Work out the finished part from the listing and answer in its coordinate system (mm). A direction names the side the tool comes from. Coordinates: 2 decimals unless noted, no trailing zeros. Write each loop counter-clockwise with the first axis right and the second up, starting at its lowest first coordinate (ties: lowest second). Pieces come first, ordered by that corner, then holes. Notation, with made-up numbers: M 61.25,-11.5 L 100.25,-11.5 A38 cw 100.25,26.5 Z; hole C -3.75,11 d2. An arc over 180 degrees is marked long. Answer as CSV lines item,"result". Start each with the question number.
(1) A cutting plane is placed at B-B on z = -9. Give the vertices of the cut face in (x, y) (3 decimals).
(2) Find the intervals of material crossed by L1, parallel to Z at x = -135.5, y = 0.95 (3 decimals); L2, parallel to Z at x = -122.5, y = 0.25 (3 decimals); L3, parallel to X at y = 0.85, z = -173, in increasing order. Write a range as [from, to].
(3) A cutting plane is placed at D-D on y = 1.25. Count the separate pieces of the cut face and the enclosed holes in it, then the cut area to 3 significant figures.
(4) A cutting plane is placed at A-A on x = -135.5. Give the vertices of the cut face in (y, z) (3 decimals), then the cut area to 3 significant figures.
(5) The mould has two halves that part along X. Classify faces 1 (the cylindrical face through (-119.578, 0.74, -9.129)), 2 (the cylindrical face through (-135.12, 0.74, -180.4)), 3 (the cylindrical face through (-115.304, 0.76, -1.711)), 4 (the cylindrical face through (-142.696, 0.76, -202.789)): released by +X, released by -X, zero draft, split by the parting line, or undercut.
(6) A cutting plane is placed at C-C on x = -116.5. Give the vertices of the cut face in (y, z).
(7) For faces 5 (the cylindrical face through (-132.578, 0.74, -27.129)), 6 (the cylindrical face through (-115.211, 0.76, -16.196)), determine the directions among +Z, -Z, +X, -X, +Y, -Y from which every point of the face is accessible in a straight line to the end or side of a thin tool.
(8) A flat-ended cylindrical pin translates along its axis: P1, Ø7.5, axis at x = -122.5, z = -195.5, coming from the +Y side. Find the tip coordinate at first contact, or state that the pin passes through.
Autodesk Inventor part; units mm, degrees
ref_plane "YZ Plane" through (0, 0, 0) normal (1, 0, 0) x (0, 1, 0)
ref_plane "XZ Plane" through (0, 0, 0) normal (0, 1, 0) x (-1, 0, 0)
ref_plane "XY Plane" through (0, 0, 0) normal (0, 0, 1) x (1, 0, 0)
sketch "Sketch1" plane through (0, 0, 0) normal (0, 1, 0) x (-1, 0, 0)
  line L0 (0, 0) -> (144.5, 0) construction
  line L1 (144.5, 0) -> (144.5, -204.5) construction
  line L2 (144.5, -204.5) -> (0, -204.5) construction
  line L3 (0, -204.5) -> (0, 0) construction
  circle A0 centre (135.5, -27) radius 3 construction
  circle A1 centre (122.5, -9) radius 3 construction
  circle A2 centre (135.5, -177.5) radius 3 construction
  circle A3 centre (122.5, -195.5) radius 3 construction
  circle A4 centre (22, -195.5) radius 3 construction
  circle A5 centre (9, -177.5) radius 3 construction
  circle A6 centre (9, -27) radius 3 construction
  circle A7 centre (22, -9) radius 3 construction
  line L4 (12, -12) -> (132.5, -12) construction
  line L5 (132.5, -12) -> (132.5, -192.5) construction
  line L6 (132.5, -192.5) -> (12, -192.5) construction
  line L7 (12, -192.5) -> (12, -12) construction
  circle A8 centre (22, -9) radius 2.925
  circle A9 centre (9, -27) radius 2.925
  circle A10 centre (122.5, -9) radius 2.925
  circle A11 centre (135.5, -27) radius 2.925
  circle A12 centre (135.5, -177.5) radius 2.925
  circle A13 centre (122.5, -195.5) radius 2.925
  circle A14 centre (22, -195.5) radius 2.925
  circle A15 centre (9, -177.5) radius 2.925
  line L8 (122.5, -9) -> (135.5, -9) construction
  line L9 (135.5, -9) -> (135.5, -27) construction
  line L10 (126.5, -27) -> (126.5, -18)
  line L11 (126.5, -18) -> (122.5, -18)
  line L12 (144.5, -27) -> (144.5, 0)
  line L13 (144.5, 0) -> (122.5, 0)
  line L14 (122.5, -195.5) -> (135.5, -195.5) construction
  line L15 (135.5, -195.5) -> (135.5, -177.5) construction
  line L16 (126.5, -177.5) -> (126.5, -186.5)
  line L17 (126.5, -186.5) -> (122.5, -186.5)
  line L18 (144.5, -177.5) -> (144.5, -204.5)
  line L19 (144.5, -204.5) -> (122.5, -204.5)
  line L20 (126.5, -27) -> (126.5, -177.5)
  line L21 (144.5, -177.5) -> (144.5, -27)
  line L22 (122.5, -9) -> (113.5, -9) construction
  line L23 (122.5, 0) -> (113.5, 0)
  line L24 (122.5, -18) -> (113.5, -18)
  line L25 (113.5, -18) -> (113.5, 0)
  line L26 (122.5, -195.5) -> (113.5, -195.5) construction
  line L27 (122.5, -204.5) -> (113.5, -204.5)
  line L28 (122.5, -186.5) -> (113.5, -186.5)
  line L29 (113.5, -186.5) -> (113.5, -204.5)
  line L30 (75.275, -87.25) -> (69.225, -87.25) construction
  line L31 (69.225, -87.25) -> (69.225, -117.25) construction
  line L32 (69.225, -117.25) -> (75.275, -117.25) construction
  line L33 (75.275, -117.25) -> (75.275, -87.25) construction
  line L34 (75.185, -87.75) -> (73.8621, -87.75)
  line L35 (69.315, -87.75) -> (69.315, -91.25)
  line L36 (69.315, -116.75) -> (70.6379, -116.75)
  line L37 (75.185, -116.75) -> (75.185, -113.25)
  arc A16 (73.8621, -116.75) -> (75.185, -113.25) centre (75.185, -115.25) ccw
  arc A17 (69.315, -113.25) -> (70.6379, -116.75) centre (69.315, -115.25) ccw
  arc A18 (75.185, -91.25) -> (73.8621, -87.75) centre (75.185, -89.25) ccw
  arc A19 (70.6379, -87.75) -> (69.315, -91.25) centre (69.315, -89.25) ccw
  line L38 (69.315, -91.25) -> (69.315, -113.25)
  line L39 (70.6379, -87.75) -> (69.315, -87.75)
  line L40 (73.8621, -87.75) -> (70.6379, -87.75)
  line L41 (75.185, -91.25) -> (75.185, -87.75)
  line L42 (75.185, -113.25) -> (75.185, -91.25)
  line L43 (70.6379, -116.75) -> (73.8621, -116.75)
  line L44 (73.8621, -116.75) -> (75.185, -116.75)
  line L45 (69.315, -113.25) -> (69.315, -116.75)
  arc A20 (69.315, -91.25) -> (70.6379, -87.75) centre (69.315, -89.25) ccw
  arc A21 (73.8621, -87.75) -> (75.185, -91.25) centre (75.185, -89.25) ccw
  arc A22 (75.185, -113.25) -> (73.8621, -116.75) centre (75.185, -115.25) ccw
  arc A23 (70.6379, -116.75) -> (69.315, -113.25) centre (69.315, -115.25) ccw
  point P0 (132.5, -102.25)
  point P1 (144.5, -102.25)
  point P2 (72.25, -12)
  point P3 (72.25, 0)
  point P4 (72.25, -87.25)
  point P5 (75.275, -102.25)
  point P6 (75.185, -102.25)
  point P7 (72.25, -87.75)
  point P8 (75.185, -102.25)
  point P9 (72.25, -87.75)
  dimension "d0" = 144.5
  dimension "d1" = 204.5
  dimension "d2" = 6
  dimension "d3" = 6
  dimension "d4" = 6
  dimension "d5" = 6
  dimension "d6" = 6
  dimension "d7" = 6
  dimension "d8" = 6
  dimension "d9" = 6
  dimension "d10" = 120.5
  dimension "d11" = 180.5
  dimension "d12" = 15
  dimension "d13" = 10
  dimension "d14" = 10
  dimension "d15" = 15
  dimension "d16" = 15
  dimension "d17" = 10
  dimension "d18" = 10
  dimension "d19" = 15
  dimension "d20" = 0.075
  dimension "d21" = 0.075
  dimension "d22" = 0.075
  dimension "d23" = 0.075
  dimension "d24" = 0.075
  dimension "d25" = 0.075
  dimension "d26" = 0.075
  dimension "d27" = 0.075
  dimension "d28" = 9
  dimension "d29" = 9
  dimension "d30" = 9
  dimension "d31" = 9
  dimension "d32" = 9
  dimension "d33" = 9
  dimension "pcbH" = 6.05
  dimension "pcbW" = 30
  dimension "pcbWcut" = 29
  dimension "pcbHcut" = 5.87
  dimension "clearance" = 4
  dimension "d42" = 1.5
  dimension "d43" = 4
  dimension "d44" = 1.5
  dimension "d45" = 1.5
  dimension "d46" = 1.5
  dimension "d47" = 4
  dimension "d48" = 4
extrude "Extrusion1" add sketch "Sketch1" along normal blind 1.5 contours L10 L11 L24 L25 L23 L13 L12 L21 L18 L19 L27 L29 L28 L17 L16 L20
fillet "Fillet1" radius 6 8 edges at (-144.5, 0.75, 0) (-113.5, 0.75, 0) (-113.5, 0.75, -18) (-126.5, 0.75, -18) (-126.5, 0.75, -186.5) (-113.5, 0.75, -186.5) (-113.5, 0.75, -204.5) (-144.5, 0.75, -204.5)
equation "\"d0\" = height"
equation "\"d1\" = width"
equation "\"d2\" = pinD"
equation "\"d3\" = pinD"
equation "\"d4\" = pinD"
equation "\"d5\" = pinD"
equation "\"d6\" = pinD"
equation "\"d7\" = pinD"
equation "\"d8\" = pinD"
equation "\"d9\" = pinD"
equation "\"d10\" = stencilH"
equation "\"d11\" = stencilW"
equation "\"d12\" = cornerW"
equation "\"d13\" = cornerH"
equation "\"d14\" = cornerH"
equation "\"d15\" = cornerW"
equation "\"d16\" = cornerW"
equation "\"d17\" = cornerH"
equation "\"d18\" = cornerH"
equation "\"d19\" = cornerW"
equation "\"d20\" = kerf"
equation "\"d21\" = kerf"
equation "\"d22\" = kerf"
equation "\"d23\" = kerf"
equation "\"d24\" = kerf"
equation "\"d25\" = kerf"
equation "\"d26\" = kerf"
equation "\"d27\" = kerf"
equation "\"d28\" = 1.5 * pinD"
equation "\"d29\" = 1.5 * pinD"
equation "\"d30\" = 1.5 * pinD"
equation "\"d31\" = 1.5 * pinD"
equation "\"d32\" = 1.5 * pinD"
equation "\"d33\" = 1.5 * pinD"
equation "\"d43\" = clearance"
equation "\"d44\" = d42"
equation "\"d45\" = d42"
equation "\"d46\" = d45"
equation "\"d47\" = clearance"
equation "\"d48\" = clearance"
equation "\"d36\" = pinD"
properties part number "side"
Here are the results:
1,outline,"M -144.5,0 L -125.425,0 L -125.425,1.5 L -144.5,1.5 Z; M -119.575,0 L -113.5,0 L -113.5,1.5 L -119.575,1.5 Z"
2,L1,"z = [-204.5, -180.425], [-174.575, -29.925], [-24.075, 0]"
2,L2,"z = [-204.5, -198.425], [-192.575, -186.157], [-18.343, -11.925], [-6.075, 0]"
2,L3,"x = [-144.5, -126.5]"
3,separate pieces,"1"
3,enclosed holes,"4"
3,area,"4,010 mm^2"
4,outline,"M 0,-204.5 L 1.5,-204.5 L 1.5,-180.425 L 0,-180.425 Z; M 0,-174.575 L 1.5,-174.575 L 1.5,-29.925 L 0,-29.925 Z; M 0,-24.075 L 1.5,-24.075 L 1.5,0 L 0,0 Z"
4,area,"289 mm^2"
5,face 1,"undercut"
5,face 2,"undercut"
5,face 3,"released by +X"
5,face 4,"released by -X"
6,outline,"M 0,-203.7 L 1.5,-203.7 L 1.5,-187.3 L 0,-187.3 Z; M 0,-17.2 L 1.5,-17.2 L 1.5,-0.8 L 0,-0.8 Z"
7,face 5,"+Y, -Y"
7,face 6,"+X, +Y, -Y"
8,P1,"stops at y = 1.5"
